```python
from build123d import *

# Parameters (mm, degrees)
SALIENTE_EXTRUIR1_DEPTH = 8


with BuildPart() as part:
    # Croquis3 → Saliente-Extruir1 (new body)
    with BuildSketch(Plane.XY):
        with BuildLine():
            Line((10, 100), (10, 0))
            ThreePointArc((10, 0), (0, -10), (-10, 0))
            Line((-10, 0), (-10, 100))
            ThreePointArc((-10, 100), (0, 110), (10, 100))
        make_face()
        with BuildLine():
            ThreePointArc((-1.428285686, 1.4), (0, -2), (1.428285686, 1.4))
            Line((1.428285686, 1.4), (-1.428285686, 1.4))
        make_face(mode=Mode.SUBTRACT)
    extrude(amount=SALIENTE_EXTRUIR1_DEPTH)


solid = part.part
```
Design review of the part built by this model. Coordinates are the model's own, in mm. Coordinates: 2 decimals unless noted, no trailing zeros. Loops run counter-clockwise (first coordinate to the right, second up) from the corner with the lowest first, then second, coordinate; pieces in that order, holes last.
Q1. We need section A-A on x = 0. State the section outline as (y, z) points, and give its area (3 significant figures).
Reported:
outline: (-10, 0) - (-2, 0) - (-2, 8) - (-10, 8) - close; (1.4, 0) - (110, 0) - (110, 8) - (1.4, 8) - close
area: 933 mm2
Q2. We need section B-B on z = 6. State the section outline as (x, y) points, and give its area (3 significant figures).
Reported:
outline: (-10, 0) arc R10 ccw to (10, 0) - (10, 100) arc R10 ccw to (-10, 100) - close; hole (-1.43, 1.4) arc R2 ccw (long way) to (1.43, 1.4) - close
area: 2,300 mm2
Q3. We need section D-D on x = -5. State the section outline as (y, z) points.
Reported:
outline: (-8.66, 0) - (108.66, 0) - (108.66, 8) - (-8.66, 8) - close
Q4. The part is to be moulded in two halves that separate along X. For faces 1 (the face through (0, 51, 0)), 2 (the face through (0, -2, 4)), 3 (the face through (0, 1.4, 4)), 4 (the face through (0, 110, 4)), say which applies: +X half, -X half, draft (parallel to the pull), parting line (faces both ways), or undercut.
Reported:
face 1: draft
face 2: undercut
face 3: undercut
face 4: parting line
Q5. To check wall thickness, follow line 1 (X direction, y = 0, z = 4.5); line 2 (Y direction, x = 0, z = 5.75); line 3 (Y direction, x = 7.5, z = 7). State the ranges of each line that lie inside material, in increasing order.
Reported:
line 1: x = -10 to -2, 2 to 10
line 2: y = -10 to -2, 1.4 to 110
line 3: y = -6.61 to 106.61
Q6. We need section C-C on x = 8.75. State the section outline as (y, z) points.
Reported:
outline: (-4.84, 0) - (104.84, 0) - (104.84, 8) - (-4.84, 8) - close
